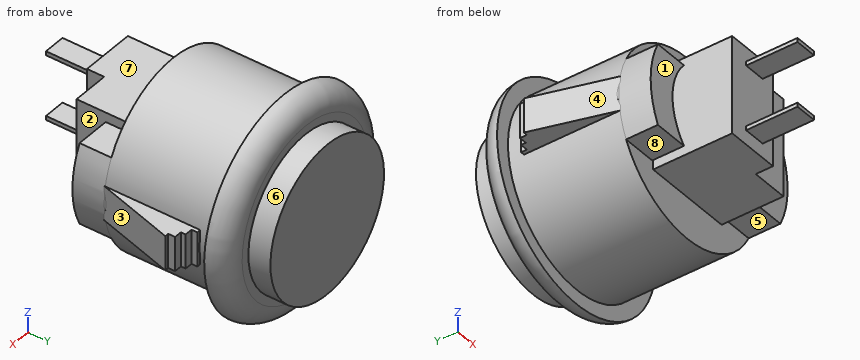
from build123d import *

# Parameters (mm, degrees)
BOSS_EXTRUDE1_DEPTH   = 6.33
BOSS_EXTRUDE2_DEPTH   = 4.11
SKETCH4_W             = 2.83
SKETCH4_H             = 0.53
BOSS_EXTRUDE3_DEPTH   = 6.65
BOSS_EXTRUDE4_DEPTH   = 2.225
BOSS_EXTRUDE4_2_DEPTH = 2.225


with BuildPart() as part:
    # Sketch1 → Revolve1 (revolve)
    with BuildSketch(Plane.XY, mode=Mode.PRIVATE) as revolve1_sk:
        with BuildLine():
            Line((0, 0), (-11.75, 0))
            Line((-11.75, 0), (-11.75, 14.35))
            Line((-11.75, 14.35), (-13.625, 14.35))
            ThreePointArc((-13.625, 14.35), (-12.804898987, 16.329898987), (-10.825, 17.15))
            Line((-10.825, 17.15), (-9.75, 17.15))
            Line((-9.75, 17.15), (-9.75, 20))
            Line((-9.75, 20), (0, 20))
            Line((0, 20), (0, 0))
        make_face()
    revolve(revolve1_sk.sketch.rotate(Axis((0, 0, 0), (0, -1, 0)), 270), axis=Axis((0, 0, 0), (0, -1, 0)))

    # Sketch2 → Boss-Extrude1 (add, symmetric)
    with BuildSketch(Plane.XY):
        Polygon((-5.875, 0), (-5.875, -10.23), (1.125, -10.23), (1.125, -8), (5.875, -8), (5.875, 0), align=None)
    extrude(amount=BOSS_EXTRUDE1_DEPTH, both=True)

    # Sketch3 → Boss-Extrude2 (add)
    with BuildSketch(Plane.XZ):
        with BuildLine():
            Line((-10.511898021, 5.25), (-6.036348234, 5.25))
            ThreePointArc((-6.036348234, 5.25), (-8, 0), (-6.036348234, -5.25))
            Line((-6.036348234, -5.25), (-10.511898021, -5.25))
            ThreePointArc((-10.511898021, -5.25), (-11.75, 0), (-10.511898021, 5.25))
        make_face()
        with BuildLine():
            Line((10.511898021, -5.25), (6.036348234, -5.25))
            ThreePointArc((6.036348234, -5.25), (8, 0), (6.036348234, 5.25))
            Line((6.036348234, 5.25), (10.511898021, 5.25))
            ThreePointArc((10.511898021, 5.25), (11.75, 0), (10.511898021, -5.25))
        make_face()
    extrude(amount=BOSS_EXTRUDE2_DEPTH)

    # Sketch4 → Boss-Extrude3 (add)
    with BuildSketch(Plane.XZ.offset(10.23)):
        with Locations((-2.07, 4.21)):
            Rectangle(SKETCH4_W, SKETCH4_H)
        with Locations((-2.07, -4.21)):
            Rectangle(SKETCH4_W, SKETCH4_H)
    extrude(amount=BOSS_EXTRUDE3_DEPTH)


with BuildPart() as body_2:
    # Sketch5 → Boss-Extrude4 (new, symmetric)
    with BuildSketch(Plane.XY):
        Polygon((-11.65, -0.11), (-14.65, 10.1), (-14.15, 10.1), (-14.15, 10.99), (-13.15, 10.99), (-13.15, 11.6), (-12.15, 11.6), (-12.15, 12.35), (-11.65, 12.35), align=None)
    extrude(amount=BOSS_EXTRUDE4_DEPTH, both=True)


with BuildPart() as body_3:
    # Sketch5 → Boss-Extrude4 2 (new, symmetric)
    with BuildSketch(Plane.XY):
        Polygon((11.65, 12.35), (11.65, -0.11), (14.65, 10.1), (14.15, 10.1), (14.15, 10.99), (13.15, 10.99), (13.15, 11.6), (12.15, 11.6), (12.15, 12.35), align=None)
    extrude(amount=BOSS_EXTRUDE4_2_DEPTH, both=True)

    # Combine2: union body 2, part
    add(body_2.part)
    add(part.part)


solid = body_3.part
Could you check a few things on this model? Use its own coordinates, in mm. Face numbers are marked on the shaded views. A direction names the side the tool comes from. Give positions to 0.01 mm unless a question says otherwise; leave off trailing zeros. Order: outer loops, then holes, each group sorted by start corner. A loop starts at its lowest first (then second) coordinate and runs counter-clockwise, first axis right, second up. Notation, with made-up numbers: (-39, 73.25) -> (-27, 73.25) arc R35 cw to (-27, 107.25) -> close; hole circle Ø3 at (-16, -22). An arc over 180 degrees is marked (long way). Return JSON: item names as keys, results as strings.
1. For pin 1 Ø3 at (x, y) = (-2.5, -13) entering from +Z (3 decimals); pin 2 Ø0.7 at (y, z) = (11.5, 0.5) entering from +X; pin 3 Ø0.6 at (y, z) = (4, -2) entering from -X, each with a flat end and sliding along its axis, tell me the tip position at first contact or that it passes through.
Answer list:
{"pin 1": "stops at z = 4.475", "pin 2": "stops at x = 13.15", "pin 3": "stops at x = -12.95"}
2. Imagine slicing it at A-A on x = 0. List the corners of the cut face in (y, z) for me (3 decimals), then the cut area to 3 significant figures.
Answer list:
{"outline": "(-10.23, -6.33) -> (0, -6.33) -> (0, -11.75) -> (14.35, -11.75) -> (14.35, -13.625) arc R2.8 ccw to (17.15, -10.825) -> (17.15, -9.75) -> (20, -9.75) -> (20, 9.75) -> (17.15, 9.75) -> (17.15, 10.825) arc R2.8 ccw to (14.35, 13.625) -> (14.35, 11.75) -> (0, 11.75) -> (0, 6.33) -> (-10.23, 6.33) -> close", "area": "595 mm2"}
3. I need wall thicknesses on line 1 (X direction, y = -2, z = -1.75) (3 decimals); line 2 (Y direction, x = 5, z = 4); line 3 (Y direction, x = 5.5, z = 7). Which ranges of each line are inside material? Lowest first, please. Write a range as from..to.
Answer list:
{"line 1": "x = -11.619..-7.806, -5.875..5.875, 7.806..11.619", "line 2": "y = -8..20", "line 3": "y = 0..20"}
4. Imagine slicing it at B-B on y = -5. List the corners of the cut face in (x, z) for me (3 decimals), then the cut area to 3 significant figures.
Answer list:
{"outline": "(-5.875, -6.33) -> (5.875, -6.33) -> (5.875, 6.33) -> (-5.875, 6.33) -> close", "area": "149 mm2"}
5. Thinking about a two-plate mould opening in X: for the marked faces 1, 2, 3 and 4, which applies, pulls with the +X half, pulls with the -X half, needs draft (parallel to the pull), parting line crosses it, or undercut?
Answer list:
{"face 1": "needs draft", "face 2": "undercut", "face 3": "pulls with the +X half", "face 4": "pulls with the -X half"}
6. On a 3-axis mill with a long thin cutter (end or side, diameter ignored), from which of +Z, -Z, +X, -X, +Y, -Y can I reach the whole of each face in a straight line? I mean the marked faces 5, 6, 7 and 8. Say none if no direction works.
Answer list:
{"face 5": "-Z, +X, -Y", "face 6": "+Y", "face 7": "+Z, +X, -X, -Y", "face 8": "-Z, -X, -Y"}
